Part model, mm, in its own coordinate system. A direction names the side the tool comes from. Give positions to 0.01 mm unless a question says otherwise; leave off trailing zeros. Write item = value, one per line. Start each with the question number.
Item 1: Tool access for faces 5 (the face through (-5.69, -37.686, -31.878)), 6 (the face through (-34.925, -34, -17)): list every direction of +Z, -Z, +X, -X, +Y, -Y with a clear straight run to the whole face (end or side of a thin tool).
Item 2: Pull direction Y, two halves, no side cores. Call faces 1 (the face through (-42.922, -1.449, -38.056)), 2 (the face through (-40.63, -6.046, -38.056)), 3 (the face through (41.2, -4.6, -38.1)), 4 (the face through (-43.001, -74.672, -38.056)): +Y half, -Y half, draft (parallel to the pull), parting line (faces both ways), or undercut.
Item 3: Drill centre lines: line 1 along Y through (x, z) = (-39, -39); line 2 along Z through (x, y) = (36.5, -52) (3 decimals); line 3 along Z through (x, y) = (-1.5, -11) (3 decimals). Where is each one in solid material? Low to high.
Item 4: Flat gauge pins, fed straight in: P1, Ø12, axis at y = -15.5, z = 8.5, coming from the -X side; P2, Ø3, axis at y = -49, z = 23.5, coming from the -X side; P3, Ø12, axis at y = -67.5, z = 26.5, coming from the -X side; P4, Ø10, axis at x = -13.5, z = -15.5, coming from the -Y side. Where does each tip first touch, or does it go through?
```python
from build123d import *

# Parameters (mm, degrees)
F1_DEPTH  = 76.2
F3_DEPTH  = 69.851
F6_DEPTH  = 76.2
F4_R      = 26.25
F7_DEPTH  = 76.1115745433
F8_R      = 6.35
F9_R      = 5.08
F10_R     = 1.5875
F11_DEPTH = 25.4


with BuildPart() as f1:
    # F0 (on Front) → F1 (new body)
    with BuildSketch(Plane.XZ):
        with BuildLine():
            Line((-34.925, -34.925), (34.925, -34.925))
            Line((34.925, -34.925), (34.925, 0))
            ThreePointArc((34.925, 0), (0, 34.925), (-34.925, 0))
            Line((-34.925, 0), (-34.925, -34.925))
        make_face()
    extrude(amount=F1_DEPTH)

    # F2 (on face) → F3 (cut, through all)
    with BuildSketch(Plane.YZ.offset(34.925)):
        Polygon((-76.2, 35.1284742355), (-76.2, -34.925), (-63.5, 35.1284742355), align=None)
    extrude(amount=-F3_DEPTH, mode=Mode.SUBTRACT)

    # F5 (on face) → F6 (join)
    with BuildSketch(Plane(origin=(0, 0, 0), x_dir=(-1, 0, 0), z_dir=(0, 1, 0))):
        Polygon((-34.925, -34.925), (-44.45, -34.925), (-44.45, -41.275), (44.45, -41.275), (44.45, -34.925), (34.925, -34.925), align=None)
    extrude(amount=-F6_DEPTH)

    # F4 (on face) → F7 (cut, through all)
    with BuildSketch(Plane(origin=(0, -67.6452101377, 12.2634056073), x_dir=(1, 0, 0), z_dir=(0, -0.9839612366, 0.178382412))):
        with Locations((0, -12.4633015524)):
            Circle(F4_R)
    extrude(amount=-F7_DEPTH, mode=Mode.SUBTRACT)

    # F8
    f8_edges = [f1.edges().sort_by_distance(p)[0] for p in [
        (0, -63.536888, 34.925),
    ]]
    fillet(f8_edges, radius=F8_R)

    # F9
    f9_edges = [f1.edges().sort_by_distance(p)[0] for p in [
        (-44.45, -76.2, -38.1),
        (-44.45, 0, -38.1),
        (44.45, -76.2, -38.1),
        (44.45, 0, -38.1),
    ]]
    fillet(f9_edges, radius=F9_R)

    # F10 (on face) → F11 (cut)
    with BuildSketch(Plane.XY.offset(-34.925)):
        with Locations((-39.37, -5.08)):
            Circle(F10_R)
        with Locations((-39.37, -68.58)):
            Circle(F10_R)
        with Locations((39.6875, -68.58)):
            Circle(F10_R)
        with Locations((39.6875, -5.08)):
            Circle(F10_R)
    extrude(amount=-F11_DEPTH, mode=Mode.SUBTRACT)


solid = f1.part
```
Values found:
q1.face_5 = none
q1.face_6 = +Z, -X, +Y, -Y
q2.face_1 = +Y half
q2.face_2 = undercut
q2.face_3 = undercut
q2.face_4 = -Y half
q3.line_1 = -76.2 to -70.12, -67.04 to -6.62, -3.54 to 0
q3.line_2 = -41.275 to -34.925
q3.line_3 = -41.275 to -37.307, 15.962 to 34.893
q4.P1 = -34.84
q4.P2 = -27.12
q4.P3 = -25.8
q4.P4 = through
